Can you work these out from the model? Positions are in its coordinate system, mm. Face numbers are marked on the shaded views. Coordinates: 2 decimals unless noted, no trailing zeros. Order: outer loops, then holes, each group sorted by start corner. A loop starts at its lowest first (then second) coordinate and runs counter-clockwise, first axis right, second up. Notation, with made-up numbers: M -34.75,87 L 7.25,87 A11 cw 7.25,101 Z; hole C 18,57.25 d2. An arc over 180 degrees is marked long. Answer as a JSON object with one key per item and string values.
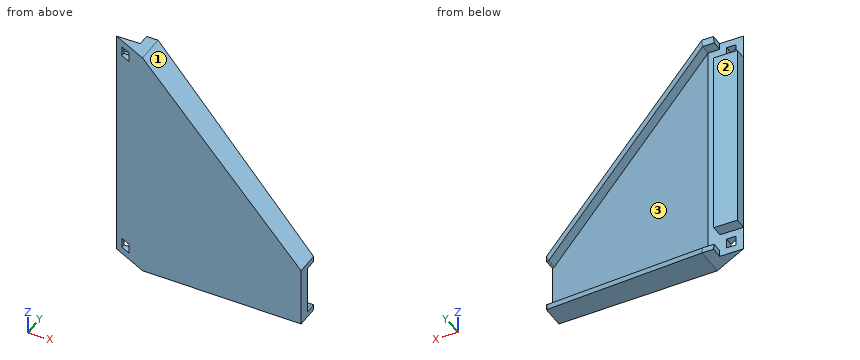
from build123d import *

# Parameters (mm, degrees)
SALIENTE_EXTRUIR1_DEPTH  = 200
CROQUIS2_W               = 8.2
CROQUIS2_H               = 8.2
CORTAR_EXTRUIR1_DEPTH    = 200
CORTAR_EXTRUIR3_DEPTH    = 313.49262378
SALIENTE_EXTRUIR3_DEPTH  = 5
SALIENTE_EXTRUIR4_REACH  = 313.287
CROQUIS10_W              = 4.621603975
CROQUIS10_H              = 10
CROQUIS11_W              = 20
CROQUIS11_H              = 159.6
SALIENTE_EXTRUIR6_DEPTH  = 10
CORTAR_EXTRUIR4_DEPTH    = 313.49262378
SALIENTE_EXTRUIR10_REACH = 299.92


with BuildPart() as part:
    # Croquis1 → Saliente-Extruir1 (new body)
    with BuildSketch(Plane.XY):
        Polygon((4.273004903, 100), (215.932026149, -5), (215.932026149, 5), (34.273004903, 100), align=None)
    extrude(amount=SALIENTE_EXTRUIR1_DEPTH)

    # Croquis2 → Cortar-Extruir1 (cut)
    with BuildSketch(Plane(origin=(0, 100, 0), x_dir=(1, 0, 0), z_dir=(0, 1, 0))):
        with Locations((14.623004903, -10)):
            Rectangle(CROQUIS2_W, CROQUIS2_H)
    cortar_extruir1 = extrude(amount=-CORTAR_EXTRUIR1_DEPTH, mode=Mode.SUBTRACT)

    # Croquis8 → Cortar-Extruir3 (cut, through all)
    with BuildSketch(Plane(origin=(0, 100, 0), x_dir=(1, 0, 0), z_dir=(0, 1, 0))):
        Polygon((34.273004903, -200), (215.932026149, -200), (215.932026149, -125), align=None)
        Polygon((215.932026149, -75), (215.932026149, 0), (34.273004903, 0), align=None)
    extrude(amount=-CORTAR_EXTRUIR3_DEPTH, mode=Mode.SUBTRACT)

    # Croquis9 → Saliente-Extruir3 (add)
    with BuildSketch(Plane(origin=(4.991214306, 0, -12.08932141), x_dir=(-0.9243207949834489, 0, -0.3816163884860884), z_dir=(0.38161638848608836, 0, -0.9243207949834488))):
        Polygon((-228.211691209, 5), (-228.211691209, 15), (-31.679251139, 110), (-31.679251139, 100), align=None)
    saliente_extruir3 = extrude(amount=-SALIENTE_EXTRUIR3_DEPTH)

    # Simetría2: Saliente-Extruir3 across plane
    add(saliente_extruir3.mirror(Plane.XY.offset(100)))

    # Croquis10 → Saliente-Extruir4 (add, up to next)
    with BuildSketch(Plane(origin=(215.932026149, 0, 0), x_dir=(0, 0, -1), z_dir=(1, 0, 0)), mode=Mode.PRIVATE) as saliente_extruir4_sk1:
        with Locations((-122.689198013, 10)):
            Rectangle(CROQUIS10_W, CROQUIS10_H)
    saliente_extruir4_tool1 = extrude(saliente_extruir4_sk1.sketch, amount=-SALIENTE_EXTRUIR4_REACH, mode=Mode.PRIVATE) - part.part
    # Croquis10 → Saliente-Extruir4 (add, up to next)
    with BuildSketch(Plane(origin=(215.932026149, 0, 0), x_dir=(0, 0, -1), z_dir=(1, 0, 0)), mode=Mode.PRIVATE) as saliente_extruir4_sk2:
        with Locations((-77.310801987, 10)):
            Rectangle(CROQUIS10_W, CROQUIS10_H)
    saliente_extruir4_tool2 = extrude(saliente_extruir4_sk2.sketch, amount=-SALIENTE_EXTRUIR4_REACH, mode=Mode.PRIVATE) - part.part
    add(saliente_extruir4_tool1.solids().sort_by_distance((215.932026, 10, 122.689198))[0])
    add(saliente_extruir4_tool2.solids().sort_by_distance((215.932026, 10, 77.310802))[0])

    # Croquis11 → Saliente-Extruir6 (add)
    with BuildSketch(Plane(origin=(0, 100, 0), x_dir=(1, 0, 0), z_dir=(0, 1, 0))):
        with Locations((14.273004903, -100)):
            Rectangle(CROQUIS11_W, CROQUIS11_H)
    extrude(amount=SALIENTE_EXTRUIR6_DEPTH)

    # Croquis12 → Cortar-Extruir4 (cut, through all)
    with BuildSketch(Plane(origin=(0, 100, 0), x_dir=(1, 0, 0), z_dir=(0, 1, 0))):
        Polygon((34.273004903, -200), (34.273004903, -194.59062262), (32.364922961, -195.378396025), align=None)
    cortar_extruir4 = extrude(amount=CORTAR_EXTRUIR4_DEPTH, mode=Mode.SUBTRACT)

    # Simetría3: Cortar-Extruir4 across plane
    add(cortar_extruir4.mirror(Plane.XY.offset(100)), mode=Mode.SUBTRACT)

    # Simetría5: Cortar-Extruir1 across plane
    add(cortar_extruir1.mirror(Plane.XY.offset(100)), mode=Mode.SUBTRACT)

    # Croquis17 → Saliente-Extruir10 (add, up to next)
    with BuildSketch(Plane.ZY.offset(-24.473004903), mode=Mode.PRIVATE) as saliente_extruir10_sk1:
        Polygon((194.59062262, 109.002153687), (194.59062262, 100), (200, 100), (200, 110), align=None)
    saliente_extruir10_tool1 = extrude(saliente_extruir10_sk1.sketch, amount=-SALIENTE_EXTRUIR10_REACH, mode=Mode.PRIVATE) - part.part
    saliente_extruir10 = saliente_extruir10_tool1.solids().sort_by_distance((24.473005, 104.754905, 197.342654))[0]
    add(saliente_extruir10)

    # Simetría6: Saliente-Extruir10 across plane
    add(saliente_extruir10.mirror(Plane.XY.offset(100)))


solid = part.part
Item 1: I want a section at C-C, the plane y = 33. Write out the boundary of the cut face in (x, z).
Answers follow:
{"outline": "M 139.33,43.37 L 181.51,60.79 L 179.6,65.41 L 162.39,58.3 L 162.39,141.7 L 179.6,134.59 L 181.51,139.21 L 139.33,156.63 Z"}
Item 2: Please list where these lines run through material, in increasing order: line 1 (X direction, y = 15, z = 98.5); line 2 (Y direction, x = 101, z = 80); line 3 (Y direction, x = 36.5, z = 9.5).
Answers follow:
{"line 1": "x = 175.62 to 196.81", "line 2": "y = 52.02 to 65.1", "line 3": "y = 84.01 to 98.84"}
Item 3: I want a section at D-D, the plane z = 129.5. Write out the boundary of the cut face in (x, y).
Answers follow:
{"outline": "M 4.27,100 L 205.03,0.41 L 205.03,20.7 L 191.93,26.55 L 191.93,17.55 L 34.27,100 L 24.27,100 L 24.27,110 L 4.27,110 Z"}
Item 4: I want a section at A-A, the plane z = 83. Write out the boundary of the cut face in (x, y), plus the area to 3 significant figures.
Answers follow:
{"outline": "M 4.27,100 L 215.93,-5 L 215.93,5 L 34.27,100 L 24.27,100 L 24.27,110 L 4.27,110 Z", "area": "2,680 mm^2"}
Item 5: If we mould it in two halves opening along Z, with no side actions, what happens to the marked faces 1, 2 and 3? For each: pulls with the +Z half, pulls with the -Z half, needs draft (parallel to the pull), parting line crosses it, or undercut.
Answers follow:
{"face 1": "pulls with the +Z half", "face 2": "needs draft", "face 3": "undercut"}
Item 6: I want a section at B-B, the plane x = 58. Write out the boundary of the cut face in (y, z), plus the area to 3 significant figures.
Answers follow:
{"outline": "M 73.35,9.8 L 97.59,9.8 L 96.59,15.21 L 87.59,15.21 L 87.59,184.79 L 96.59,184.79 L 97.59,190.2 L 73.35,190.2 Z", "area": "2,670 mm^2"}
Item 7: I'm going to push flat-ended pins straight in: pin 1 (6 mm diameter, centred on y = 106, z = 198, fed in from -X); pin 2 (1.5 mm diameter, centred on x = 215.5, y = 11.5, fed in from -Z); pin 3 (6 mm diameter, centred on y = 96, z = 140, fed in from +X). Where does each tip first touch, or does it pass through?
Answers follow:
{"pin 1": "stops at x = 24.47", "pin 2": "stops at z = 74.51", "pin 3": "stops at x = 47.66"}
